Model file for the job. Use its own axes, mm. A direction names the side the tool comes from. Coordinates: 2 decimals unless noted, no trailing zeros. Loops run counter-clockwise (first coordinate to the right, second up) from the corner with the lowest first, then second, coordinate; pieces in that order, holes last. Notation, with made-up numbers: (-26.5, 21) -> (-10.5, 21) arc R17 ccw to (-10.5, 29) -> close; hole circle Ø3 at (7.25, 82). An arc over 180 degrees is marked (long way). Use one line per item in the form item = value.
```python
from build123d import *

# Parameters (mm, degrees)
BOSS_EXTRUDE1_DEPTH = 1


with BuildPart() as part:
    # Sketch1 → Boss-Extrude1 (new body)
    with BuildSketch(Plane(origin=(0, 0, 0), x_dir=(1, 0, 0), z_dir=(0, 1, 0))):
        with BuildLine():
            Line((0, 3.75), (0, 1.6))
            Line((0, 1.6), (5, 1.6))
            ThreePointArc((5, 1.6), (6.6, 0), (5, -1.6))
            Line((5, -1.6), (0, -1.6))
            Line((0, -1.6), (0, -3.75))
            Line((0, -3.75), (30, -3.75))
            Line((30, -3.75), (30, 3.75))
            Line((30, 3.75), (0, 3.75))
        make_face()
    extrude(amount=BOSS_EXTRUDE1_DEPTH)


solid = part.part
```
Q1. Band-saw the part on B-B, the plane z = 0. Write the cut outline in (x, y).
Result:
outline = (6.6, 0) -> (30, 0) -> (30, 1) -> (6.6, 1) -> close
Q2. Band-saw the part on C-C, the plane z = 1.25. Write the cut outline in (x, y).
Result:
outline = (6, 0) -> (30, 0) -> (30, 1) -> (6, 1) -> close
Q3. Band-saw the part on A-A, the plane y = 0.4. Write the cut outline in (x, z), and give its area (3 significant figures).
Result:
outline = (0, -3.75) -> (30, -3.75) -> (30, 3.75) -> (0, 3.75) -> (0, 1.6) -> (5, 1.6) arc R1.6 cw to (5, -1.6) -> (0, -1.6) -> close
area = 205 mm2
Q4. Which spindle directions (+Z, -Z, +X, -X, +Y, -Y) get a long thin tool onto all of the face, cutting with end or side? Do faces 1 (the face through (30, 0.5, 0.1)), 2 (the face through (2.5, 0.5, -1.6)). Say none if no direction does.
Result:
face_1 = +Z, -Z, +X, +Y, -Y
face_2 = -X, +Y, -Y
Q5. Mould opens along Z. For faces 3 (the face through (2.5, 0.5, 1.6)), 4 (the face through (6.6, 0.5, 0)), 5 (the face through (14.8, 0.5, 3.75)), 6 (the face through (15.2, 0.5, -3.75)) say: released by +Z, released by -Z, zero draft, split by the parting line, or undercut.
Result:
face_3 = undercut
face_4 = undercut
face_5 = released by +Z
face_6 = released by -Z
Q6. Wall check: line 1 along Z through (x, y) = (4.75, 0.35); line 2 along Z through (x, y) = (6, 0.2); line 3 along X through (y, z) = (0.9, 0.5). Give the ranges that are in metal, low to high.
Result:
line_1 = -3.75 to -1.6, 1.6 to 3.75
line_2 = -3.75 to -1.25, 1.25 to 3.75
line_3 = 6.52 to 30
